The model under review builds one solid part; all positions refer to its coordinate system, in mm. Give positions to 0.01 mm unless a question says otherwise; leave off trailing zeros. Loops run counter-clockwise (first coordinate to the right, second up) from the corner with the lowest first, then second, coordinate; pieces in that order, holes last. Notation, with made-up numbers: M 2.25,-3.5 L 7.25,-3.5 A21 cw 7.25,34.5 Z; hole C -1.5,-40 d7. An arc over 180 degrees is marked long. One line per item, written item: value. Start each with the question number.
Q1. We need section C-C on x = -6.5. Write out the cut boundary in (y, z), plus the area to 3 significant figures.
Q2. We need section D-D on y = 50.8. Write out the cut boundary in (x, z), plus the area to 3 significant figures.
Q3. We need section B-B on y = -41. Write out the cut boundary in (x, z), plus the area to 3 significant figures.
Q4. We need section A-A on x = 33. Write out the cut boundary in (y, z), plus the area to 3 significant figures.
Q5. To check wall thickness, follow line 1 along Y through (x, z) = (-31.75, 0.8); line 2 along Y through (x, z) = (36.5, 0.7); line 3 along X through (y, z) = (-44, 0.15). State the ranges of each line that lie inside material, in increasing order. Write a range as from..to.
```python
from build123d import *

# Parameters (mm, degrees)
SKETCH1_W           = 128.5875
SKETCH1_H           = 144.4625
BOSS_EXTRUDE1_DEPTH = 1.21412
SKETCH3_R           = 8.73125
SKETCH3_R_2         = 19.84375
SKETCH3_W           = 79.375
SKETCH3_H           = 36.5125
SKETCH3_W_2         = 50.8
SKETCH3_H_2         = 68.2625
CUT_EXTRUDE1_DEPTH  = 2.21412
SKETCH4_W           = 50.8
SKETCH4_H           = 68.2625
SKETCH4_W_2         = 45.72
SKETCH4_H_2         = 63.1825
BOSS_EXTRUDE2_DEPTH = 1.21412
SKETCH5_W           = 79.375
SKETCH5_H           = 36.5125
SKETCH5_W_2         = 69.215
SKETCH5_H_2         = 23.8125
BOSS_EXTRUDE3_DEPTH = 1.21412


with BuildPart() as part:
    # Sketch1 → Boss-Extrude1 (new body)
    with BuildSketch(Plane.XY):
        Rectangle(SKETCH1_W, SKETCH1_H)
    extrude(amount=BOSS_EXTRUDE1_DEPTH)

    # Sketch3 → Cut-Extrude1 (cut, through all)
    with BuildSketch(Plane.XY.offset(1.21412)):
        with Locations((-31.75, 50.8)):
            Circle(SKETCH3_R)
        with Locations((-31.75, 9.525)):
            Circle(SKETCH3_R_2)
        with Locations((11.90625, -41.275)):
            Rectangle(SKETCH3_W, SKETCH3_H)
        with Locations((26.19375, 25.4)):
            Rectangle(SKETCH3_W_2, SKETCH3_H_2)
    extrude(amount=-CUT_EXTRUDE1_DEPTH, mode=Mode.SUBTRACT)

    # Sketch4 → Boss-Extrude2 (add)
    with BuildSketch(Plane.XY.offset(1.21412)):
        with Locations((26.19375, 25.4)):
            Rectangle(SKETCH4_W, SKETCH4_H)
        with Locations((26.19375, 25.4)):
            Rectangle(SKETCH4_W_2, SKETCH4_H_2, mode=Mode.SUBTRACT)
    extrude(amount=-BOSS_EXTRUDE2_DEPTH)

    # Sketch5 → Boss-Extrude3 (add)
    with BuildSketch(Plane.XY.offset(1.21412)):
        with Locations((11.90625, -41.275)):
            Rectangle(SKETCH5_W, SKETCH5_H)
        with Locations((11.90625, -41.275)):
            Rectangle(SKETCH5_W_2, SKETCH5_H_2, mode=Mode.SUBTRACT)
    extrude(amount=-BOSS_EXTRUDE3_DEPTH)


solid = part.part
```
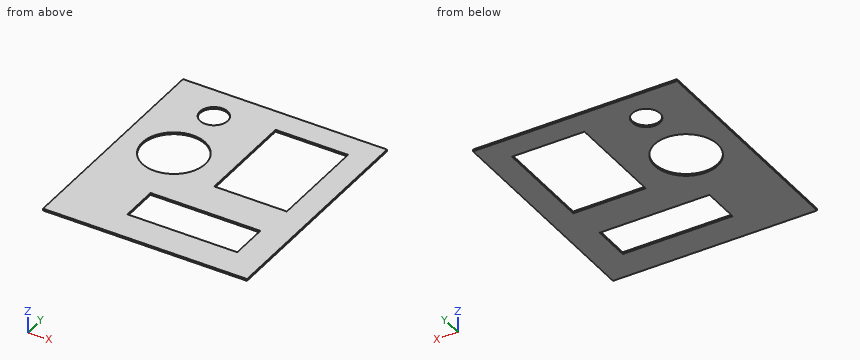
Solved:
1. outline: M -72.23,0 L -53.18,0 L -53.18,1.21 L -72.23,1.21 Z; M -29.37,0 L 72.23,0 L 72.23,1.21 L -29.37,1.21 Z
1. area: 146 mm2
2. outline: M -64.29,0 L -40.48,0 L -40.48,1.21 L -64.29,1.21 Z; M -23.02,0 L 3.33,0 L 3.33,1.21 L -23.02,1.21 Z; M 49.05,0 L 64.29,0 L 64.29,1.21 L 49.05,1.21 Z
2. area: 79.4 mm2
3. outline: M -64.29,0 L -22.7,0 L -22.7,1.21 L -64.29,1.21 Z; M 46.51,0 L 64.29,0 L 64.29,1.21 L 46.51,1.21 Z
3. area: 72.1 mm2
4. outline: M -72.23,0 L -53.18,0 L -53.18,1.21 L -72.23,1.21 Z; M -29.37,0 L -6.19,0 L -6.19,1.21 L -29.37,1.21 Z; M 56.99,0 L 72.23,0 L 72.23,1.21 L 56.99,1.21 Z
4. area: 69.8 mm2
5. line 1: -72.23..-10.32, 29.37..42.07, 59.53..72.23
5. line 2: -72.23..-53.18, -29.37..-6.19, 56.99..72.23
5. line 3: -64.29..-22.7, 46.51..64.29
